Input: part model. Units: mm. Frame: model coordinates. Face numbers are marked on the shaded views. A direction names the side the tool comes from. Coordinates: 2 decimals unless noted, no trailing zeros. Write each loop counter-clockwise with the first axis right and the second up, starting at its lowest first coordinate (ties: lowest second). Pieces come first, ordered by that corner, then holes. Notation, with made-up numbers: M 56,-13.5 L 101,-13.5 A16 ccw 101,0.5 Z; hole C 12.25,15 d10. An arc over 180 degrees is marked long. Answer as a JSON object with one key per item and string values. Group by question number.
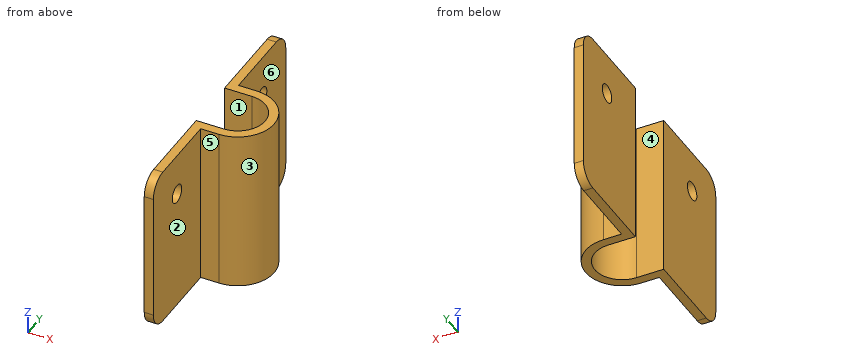
from build123d import *

# Parameters (mm, degrees)
BOSS_EXTRUDE1_DEPTH     = 88.9
SKETCH2_R               = 3.175
CUT_EXTRUDE1_DEPTH      = 4.175
FILLET1_R               = 6.35
SKETCH3_W               = 31.75
SKETCH3_H               = 57.15
CUT_EXTRUDE2_DEPTH      = 20.05
CUT_EXTRUDE2_DEPTH_BACK = 4.175
FILLET2_R               = 6.35


with BuildPart() as part:
    # Sketch1 → Boss-Extrude1 (new body)
    with BuildSketch(Plane.XY):
        with BuildLine():
            Line((13.335, 323.089397322), (10.16, 323.089397322))
            Line((10.16, 323.089397322), (10.16, 288.164397322))
            Line((10.16, 288.164397322), (19.685, 288.164397322))
            ThreePointArc((19.685, 288.164397322), (29.21, 278.639397322), (19.685, 269.114397322))
            Line((19.685, 269.114397322), (10.16, 269.114397322))
            Line((10.16, 269.114397322), (10.16, 234.189397322))
            Line((10.16, 234.189397322), (13.335, 234.189397322))
            Line((13.335, 234.189397322), (13.335, 265.939397322))
            Line((13.335, 265.939397322), (19.685, 265.939397322))
            ThreePointArc((19.685, 265.939397322), (32.385, 278.639397322), (19.685, 291.339397322))
            Line((19.685, 291.339397322), (13.335, 291.339397322))
            Line((13.335, 291.339397322), (13.335, 323.089397322))
        make_face()
    extrude(amount=-BOSS_EXTRUDE1_DEPTH)

    # Sketch2 → Cut-Extrude1 (cut, through all)
    with BuildSketch(Plane(origin=(13.335, 0, 0), x_dir=(0, 0, -1), z_dir=(1, 0, 0))):
        with Locations((46.355, 250.064397322)):
            Circle(SKETCH2_R)
        with Locations((46.355, 307.214397322)):
            Circle(SKETCH2_R)
    extrude(amount=-CUT_EXTRUDE1_DEPTH, mode=Mode.SUBTRACT)

    # Fillet1
    fillet1_edges = [part.edges().sort_by_distance(p)[0] for p in [
        (11.7475, 323.089397322, 0),
        (11.7475, 234.189397322, 0),
        (11.7475, 234.189397322, -88.9),
        (11.7475, 323.089397322, -88.9),
    ]]
    fillet(fillet1_edges, radius=FILLET1_R)

    # Sketch3 → Cut-Extrude2 (cut, two sides)
    with BuildSketch(Plane(origin=(13.335, 0, 0), x_dir=(0, 0, -1), z_dir=(1, 0, 0))) as cut_extrude2_sk:
        with Locations((15.875, 294.514397322)):
            Rectangle(SKETCH3_W, SKETCH3_H)
        with BuildLine():
            Line((31.75, 234.189397322), (31.75, 265.939397322))
            Line((31.75, 265.939397322), (0, 265.939397322))
            Line((0, 265.939397322), (0, 240.539397322))
            ThreePointArc((0, 240.539397322), (1.859871939, 236.049269261), (6.35, 234.189397322))
            Line((6.35, 234.189397322), (31.75, 234.189397322))
        make_face()
    extrude(amount=CUT_EXTRUDE2_DEPTH, mode=Mode.SUBTRACT)
    extrude(cut_extrude2_sk.sketch, amount=-CUT_EXTRUDE2_DEPTH_BACK, mode=Mode.SUBTRACT)

    # Fillet2
    fillet2_edges = [part.edges().sort_by_distance(p)[0] for p in [
        (11.7475, 234.189397322, -31.75),
        (11.7475, 323.089397322, -31.75),
    ]]
    fillet(fillet2_edges, radius=FILLET2_R)


solid = part.part
Q1. Access query for the marked faces 4, 5 and 6. Directions: +Z, -Z, +X, -X, +Y, -Y. A direction counts if a zero-diameter tool reaches every point of the face in a straight line with its end or side. Return the directions, or none.
Q2. Pin query (flat end, axial travel): pin 1 Ø12 at (y, z) = (303, -37.5) entering from +X (3 decimals); pin 2 Ø3 at (x, z) = (17, -54) entering from -Y; pin 3 Ø6 at (y, z) = (285.5, -67) entering from +X. Return the tip coordinate at first contact, or that it passes through.
Q3. Section B-B, the plane x = 16.75. Return the cut outline in (y, z), and give its area (3 significant figures).
Q4. Section D-D, the plane x = 12.25. Return the cut outline in (y, z) (3 decimals), and give its area (3 significant figures).
Q5. Section C-C, the plane y = 252. Return the cut outline in (x, z) (3 decimals), and give its area (3 significant figures).
Q6. Line query: line 1 (Y direction, x = 16.5, z = -86); line 2 (Y direction, x = 25.5, z = -84); line 3 (X direction, y = 258.5, z = -43) (3 decimals). Output: solid intervals per line, ascending. Write a range as from..to.
Q7. Draft query along Y for the marked faces 1, 2 and 3. Return one class per face: released by +Y, released by -Y, zero draft, split by the parting line, or undercut.
Q8. Section A-A, the plane z = -60. Return the cut outline in (x, y) (3 decimals).
Filled in:
{
 "1": {"face 4": "+Z, -Z, -X", "face 5": "+Z, -Z, +X, -Y", "face 6": "+Z, -Z, +X, +Y"},
 "2": {"pin 1": "x = 13.335", "pin 2": "y = 265.94", "pin 3": "x = 31.78"},
 "3": {"outline": "M 265.94,-88.9 L 269.11,-88.9 L 269.11,-31.75 L 265.94,-31.75 Z; M 288.16,-88.9 L 291.34,-88.9 L 291.34,-31.75 L 288.16,-31.75 Z", "area": "363 mm^2"},
 "4": {"outline": "M 234.189,-82.55 A6.35 ccw 240.539,-88.9 L 269.114,-88.9 L 269.114,-31.75 L 240.539,-31.75 A6.35 ccw 234.189,-38.1 Z; M 288.164,-88.9 L 316.739,-88.9 A6.35 ccw 323.089,-82.55 L 323.089,-38.1 A6.35 ccw 316.739,-31.75 L 288.164,-31.75 Z; hole C 250.064,-46.355 d6.35; hole C 307.214,-46.355 d6.35", "area": "3,890 mm^2"},
 "5": {"outline": "M 10.16,-88.9 L 13.335,-88.9 L 13.335,-48.872 L 10.16,-48.872 Z; M 10.16,-43.838 L 13.335,-43.838 L 13.335,-31.75 L 10.16,-31.75 Z", "area": "165 mm^2"},
 "6": {"line 1": "265.94..269.11, 288.16..291.34", "line 2": "267.35..271.1, 286.18..289.93", "line 3": "10.16..13.335"},
 "7": {"face 1": "undercut", "face 2": "zero draft", "face 3": "split by the parting line"},
 "8": {"outline": "M 10.16,234.189 L 13.335,234.189 L 13.335,265.939 L 19.685,265.939 A12.7 ccw 19.685,291.339 L 13.335,291.339 L 13.335,323.089 L 10.16,323.089 L 10.16,288.164 L 19.685,288.164 A9.525 cw 19.685,269.114 L 10.16,269.114 Z"}
}
